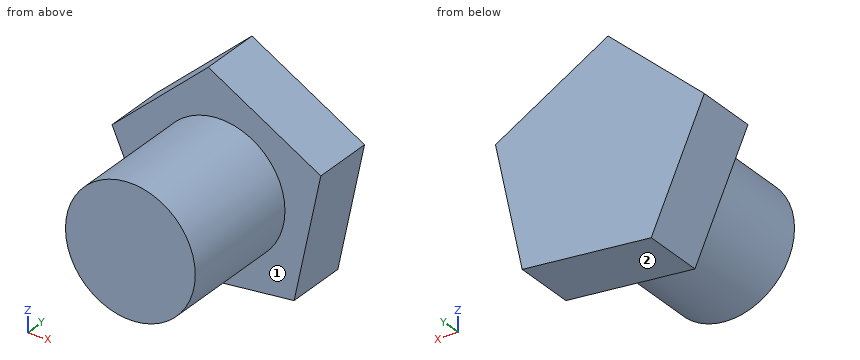
```python
from build123d import *

# Parameters (mm, degrees)
SKETCH1_R           = 5.08
BOSS_EXTRUDE1_DEPTH = 9.906
BOSS_EXTRUDE2_DEPTH = 4.826


with BuildPart() as part:
    # Sketch1 → Boss-Extrude1 (new body)
    with BuildSketch(Plane(origin=(0, 0, 0), x_dir=(1, 0, 0), z_dir=(0, 1, 0))):
        Circle(SKETCH1_R)
    extrude(amount=BOSS_EXTRUDE1_DEPTH)

    # Sketch2 → Boss-Extrude2 (add)
    with BuildSketch(Plane(origin=(0, 9.906, 0), x_dir=(1, 0, 0), z_dir=(0, 1, 0))):
        Polygon((7.887747477, -3.532447537), (5.797005266, 6.410107316), (-4.305001189, 7.49411173), (-8.457642323, -1.778491551), (-0.922109231, -8.593279957), align=None)
    extrude(amount=BOSS_EXTRUDE2_DEPTH)


solid = part.part
```
For this review, take the finished solid that the model builds, in its own axes (mm). Face numbers are marked on the shaded views. A direction names the side the tool comes from. Give positions to 0.01 mm unless a question says otherwise; leave off trailing zeros. Write each loop counter-clockwise with the first axis right and the second up, starting at its lowest first coordinate (ties: lowest second). Pieces come first, ordered by that corner, then holes. Notation, with made-up numbers: M 78.5,-12.75 L 108.5,-12.75 A30 cw 108.5,16.25 Z; hole C 24.5,-16.75 d6. An arc over 180 degrees is marked long. Answer as CSV lines item,"result".
1. Wall thickness on line 1 (Y direction, x = -1.5, z = -5); line 2 (X direction, y = 5.75, z = 2.75); line 3 (X direction, y = 4.75, z = 3.5): over which ranges is each line inside the solid? List them lowest first.
Findings:
line 1,"y = 9.91 to 14.73"
line 2,"x = -4.27 to 4.27"
line 3,"x = -3.68 to 3.68"
2. Consider section D-D, the plane y = 5. Write out the cut boundary in (x, z), then the cut area to 3 significant figures.
Findings:
outline,"C 0,0 d10.16"
area,"81.1 mm2"
3. For pin 1 (2 mm diameter, centred on y = 1.5, z = -1.5, fed in from -X); pin 2 (3 mm diameter, centred on x = -3, z = -3, fed in from -Y); pin 3 (3 mm diameter, centred on y = 9, z = -2.5, fed in from -X); pin 4 (1.5 mm diameter, centred on x = 0, y = 6, fed in from +Z), all flat-tipped, find the tip position at first contact; note any pin that passes through.
Findings:
pin 1,"stops at x = -5.06"
pin 2,"stops at y = 0"
pin 3,"stops at x = -7.08"
pin 4,"stops at z = 5.08"
4. For the marked faces 1 and 2, list the 3-axis set-ups (+Z, -Z, +X, -X, +Y, -Y) from which the entire face can be reached by the end or side of a thin tool; tool diameter is ignored.
Findings:
face 1,"-Y"
face 2,"-Z, +X, +Y, -Y"
5. Consider section C-C, the plane x = 3.5. Write out the cut boundary in (y, z), then the cut area to 3 significant figures.
Findings:
outline,"M 0,-3.68 L 9.91,-3.68 L 9.91,-6.66 L 14.73,-6.66 L 14.73,6.05 L 9.91,6.05 L 9.91,3.68 L 0,3.68 Z"
area,"134 mm2"
6. Consider section B-B, the plane z = 4.5. Write out the cut boundary in (x, y), then the cut area to 3 significant figures.
Findings:
outline,"M -5.45,9.91 L -2.36,9.91 L -2.36,0 L 2.36,0 L 2.36,9.91 L 6.2,9.91 L 6.2,14.73 L -5.45,14.73 Z"
area,"103 mm2"
7. Consider section A-A, the plane y = 12. Write out the cut boundary in (x, z) (1 decimal).
Findings:
outline,"M -8.5,1.8 L -4.3,-7.5 L 5.8,-6.4 L 7.9,3.5 L -0.9,8.6 Z"
